from build123d import *

# Parameters (mm, degrees)
SKETCH1_W           = 88
SKETCH1_H           = 91
BOSS_EXTRUDE1_DEPTH = 18
SHELL1_T            = -2
FILLET1_R           = 1
SKETCH2_R           = 2
SKETCH2_W           = 72
SKETCH2_H           = 25
CUT_EXTRUDE1_DEPTH  = 18
CUT_EXTRUDE2_REACH  = 107.256
SKETCH3_W           = 28
SKETCH3_H           = 3
SKETCH3_W_2         = 9
CUT_EXTRUDE3_REACH  = 104.367
SKETCH4_W           = 5
SKETCH4_H           = 3


with BuildPart() as part:
    # Sketch1 → Boss-Extrude1 (new body)
    with BuildSketch(Plane(origin=(0, 0, 0), x_dir=(1, 0, 0), z_dir=(0, 1, 0))):
        with Locations((-5.737068998, 3.601045098)):
            Rectangle(SKETCH1_W, SKETCH1_H)
    extrude(amount=BOSS_EXTRUDE1_DEPTH)

    # Shell1
    shell1_openings = [part.faces().sort_by_distance(p)[0] for p in [
        (-5.737068998, 0, -3.601045098),
    ]]
    offset(amount=SHELL1_T, openings=shell1_openings, kind=Kind.INTERSECTION)

    # Fillet1
    fillet1_edges = [part.edges().sort_by_distance(p)[0] for p in [
        (38.262931002, 18, -3.601045098),
        (-5.737068998, 18, -49.101045098),
        (-49.737068998, 18, -3.601045098),
        (-49.737068998, 0, -3.601045098),
        (-5.737068998, 18, 41.898954902),
        (-49.737068998, 9, -49.101045098),
        (38.262931002, 9, -49.101045098),
        (38.262931002, 9, 41.898954902),
        (-49.737068998, 9, 41.898954902),
    ]]
    fillet(fillet1_edges, radius=FILLET1_R)

    # Sketch2 → Cut-Extrude1 (cut)
    with BuildSketch(Plane(origin=(0, 18, 0), x_dir=(1, 0, 0), z_dir=(0, 1, 0))):
        with Locations(Location((-5.30968118, 1.818409631, 0), (0, 0, 270))):
            Circle(SKETCH2_R)
        with Locations(Location((-5.30968118, -8.274923211, 0), (0, 0, 270))):
            Circle(SKETCH2_R)
        with Locations(Location((-14.188721584, -3.11442221, 0), (0, 0, 270))):
            Circle(SKETCH2_R)
        with Locations(Location((3.569359225, -3.11442221, 0), (0, 0, 270))):
            Circle(SKETCH2_R)
        with Locations((-5.737068998, 26.601045098)):
            Rectangle(SKETCH2_W, SKETCH2_H)
    extrude(amount=-CUT_EXTRUDE1_DEPTH, mode=Mode.SUBTRACT)

    # Sketch3 → Cut-Extrude2 (cut, up to next)
    with BuildSketch(Plane.XY.offset(41.898954902), mode=Mode.PRIVATE) as cut_extrude2_sk1:
        with Locations((-32.237068998, 4.495374911)):
            Rectangle(SKETCH3_W, SKETCH3_H)
    cut_extrude2_tool1 = extrude(cut_extrude2_sk1.sketch, amount=-CUT_EXTRUDE2_REACH, mode=Mode.PRIVATE) & part.part
    # Sketch3 → Cut-Extrude2 (cut, up to next)
    with BuildSketch(Plane.XY.offset(41.898954902), mode=Mode.PRIVATE) as cut_extrude2_sk2:
        with Locations((20.762931002, 4.495374911)):
            Rectangle(SKETCH3_W, SKETCH3_H)
    cut_extrude2_tool2 = extrude(cut_extrude2_sk2.sketch, amount=-CUT_EXTRUDE2_REACH, mode=Mode.PRIVATE) & part.part
    # Sketch3 → Cut-Extrude2 (cut, up to next)
    with BuildSketch(Plane.XY.offset(41.898954902), mode=Mode.PRIVATE) as cut_extrude2_sk3:
        with Locations((-5.737068998, 4.495374911)):
            Rectangle(SKETCH3_W_2, SKETCH3_H)
    cut_extrude2_tool3 = extrude(cut_extrude2_sk3.sketch, amount=-CUT_EXTRUDE2_REACH, mode=Mode.PRIVATE) & part.part
    add(cut_extrude2_tool1.solids().sort_by_distance((-32.237069, 4.495375, 41.898955))[0], mode=Mode.SUBTRACT)
    add(cut_extrude2_tool2.solids().sort_by_distance((20.762931, 4.495375, 41.898955))[0], mode=Mode.SUBTRACT)
    add(cut_extrude2_tool3.solids().sort_by_distance((-5.737069, 4.495375, 41.898955))[0], mode=Mode.SUBTRACT)

    # Sketch4 → Cut-Extrude3 (cut, up to next)
    with BuildSketch(Plane(origin=(38.262931002, 0, 0), x_dir=(0, 0, -1), z_dir=(1, 0, 0)), mode=Mode.PRIVATE) as cut_extrude3_sk1:
        with Locations((0.5597151, 6.442773973)):
            Rectangle(SKETCH4_W, SKETCH4_H)
    cut_extrude3_tool1 = extrude(cut_extrude3_sk1.sketch, amount=-CUT_EXTRUDE3_REACH, mode=Mode.PRIVATE) & part.part
    add(cut_extrude3_tool1.solids().sort_by_distance((38.262931, 6.442774, -0.559715))[0], mode=Mode.SUBTRACT)


solid = part.part
Source: CAD feature listing. Evaluate the final solid. Frame: model axes, mm. A direction names the side the tool comes from. Give positions to 0.01 mm unless a question says otherwise; leave off trailing zeros. Write each loop counter-clockwise with the first axis right and the second up, starting at its lowest first coordinate (ties: lowest second). Pieces come first, ordered by that corner, then holes. Notation, with made-up numbers: (13.5, 13) -> (38.5, 13) arc R20 cw to (38.5, 52) -> close; hole circle Ø9 at (56, -37). An arc over 180 degrees is marked (long way). Return JSON: item names as keys, results as strings. Group by question number.
1. Access query for faces 1 (the face through (-32, 5.995, 41)), 2 (the face through (-6, 18, 6)), 3 (the face through (37, 7.943, -1)), 4 (the face through (38.263, 8.4, -3)), 5 (the face through (36.263, 10, -3)). Directions: +Z, -Z, +X, -X, +Y, -Y. A direction counts if a zero-diameter tool reaches every point of the face in a straight line with its end or side. Return the directions, or none.
2. Section C-C, the plane z = 7.5. Output: boundary loops of the cut face in (x, y).
3. Pin query (flat end, axial travel): pin 1 Ø5 at (x, z) = (18.5, -14) entering from -Y; pin 2 Ø2.5 at (x, z) = (-5.31, 8.27) entering from -Y. Return the tip coordinate at first contact, or that it passes through.
4. Section A-A, the plane x = 13.5. Output: boundary loops of the cut face in (y, z), then the cut area to 3 significant figures.
5. Section D-D, the plane z = 19. Output: boundary loops of the cut face in (x, y), then the cut area to 3 significant figures.
6. Material intervals for line 1 (X direction, y = 6.5, z = 26.5); line 2 (Z direction, x = -23, y = 14); line 3 (X direction, y = 16.5, z = 3.5), sorted ascending. Write a range as from..to.
7. Mould query, pull axis Y, two halves, no side actions, for faces 6 (the face through (-6, 16, 5)), 7 (the face through (-12.2, 17, 2.9)), 8 (the face through (21, 2.995, 41)). Classes: +Y half, -Y half, draft (parallel to the pull), parting line (faces both ways), or undercut.
8. Section B-B, the plane y = 12.75. Output: boundary loops of the cut face in (x, z), then the cut area to 3 significant figures.
Determined:
{
 "1": {"face 1": "+Z", "face 2": "+Z, -Z, +X, -X, +Y", "face 3": "+X", "face 4": "+Z, -Z, +X, +Y, -Y", "face 5": "-Y"},
 "2": {"outline": "(-49.74, 1) arc R1 ccw to (-48.74, 0) -> (-47.74, 0) -> (-47.74, 16) -> (-7.15, 16) -> (-7.15, 18) -> (-48.74, 18) arc R1 ccw to (-49.74, 17) -> close; (-3.47, 16) -> (36.26, 16) -> (36.26, 0) -> (38.26, 0) -> (38.26, 17) arc R1 ccw to (37.26, 18) -> (-3.47, 18) -> close"},
 "3": {"pin 1": "stops at y = 16", "pin 2": "passes through"},
 "4": {"outline": "(0, -49.1) -> (17, -49.1) arc R1 ccw to (18, -48.1) -> (18, -39.1) -> (16, -39.1) -> (16, -47.1) -> (0, -47.1) -> close; (0, 39.9) -> (3, 39.9) -> (3, 41.9) -> (0, 41.9) -> close; (6, 39.9) -> (16, 39.9) -> (16, -14.1) -> (18, -14.1) -> (18, 40.9) arc R1 ccw to (17, 41.9) -> (6, 41.9) -> close", "area": "190 mm2"},
 "5": {"outline": "(-49.74, 1) arc R1 ccw to (-48.74, 0) -> (-47.74, 0) -> (-47.74, 16) -> (36.26, 16) -> (36.26, 0) -> (38.26, 0) -> (38.26, 17) arc R1 ccw to (37.26, 18) -> (-48.74, 18) arc R1 ccw to (-49.74, 17) -> close", "area": "239 mm2"},
 "6": {"line 1": "x = -49.74..-47.74, 36.26..38.26", "line 2": "z = -49.1..-47.1, 39.9..41.9", "line 3": "x = -49.74..-16.15, -12.23..1.61, 5.53..38.26"},
 "7": {"face 6": "-Y half", "face 7": "draft", "face 8": "undercut"},
 "8": {"outline": "(-49.74, -48.1) arc R1 ccw to (-48.74, -49.1) -> (37.26, -49.1) arc R1 ccw to (38.26, -48.1) -> (38.26, 40.9) arc R1 ccw to (37.26, 41.9) -> (-48.74, 41.9) arc R1 ccw to (-49.74, 40.9) -> close; hole (-47.74, -47.1) -> (36.26, -47.1) -> (36.26, 39.9) -> (-47.74, 39.9) -> close", "area": "699 mm2"}
}
